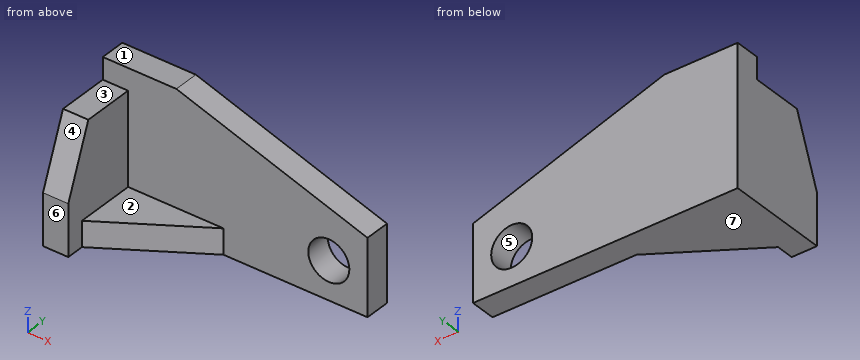
```python
from build123d import *

# Parameters (mm, degrees)
F1_DEPTH = 10.922
F3_DEPTH = 10.922
F5_DEPTH = 10.922
F6_R     = 8.859667
F7_DEPTH = 88.646


with BuildPart() as f1:
    # F0 (on Front) → F1 (new body)
    with BuildSketch(Plane.XZ):
        Polygon((31.75, 60.198), (0, 60.198), (0, 0), (114.3, 0), (114.3, 32.885686), align=None)
    extrude(amount=F1_DEPTH)

    # F2 (on Right) → F3 (join)
    with BuildSketch(Plane.YZ):
        Polygon((-44.45, 0), (0, 0), (0, 50.8), (-33.220524, 50.8), (-44.45, 22.098), align=None)
    extrude(amount=F3_DEPTH)

    # F4 (on Top) → F5 (join)
    with BuildSketch(Plane.XY):
        Polygon((52.578, -10.637136), (0, -10.637136), (0, -43.688301), align=None)
    extrude(amount=F5_DEPTH)

    # F6 (on Front) → F7 (cut)
    with BuildSketch(Plane.XZ):
        with Locations((97.587422, 16.523723)):
            Circle(F6_R)
    extrude(amount=F7_DEPTH, mode=Mode.SUBTRACT)


solid = f1.part
```
CAD build for the part. Positions are in the model's coordinates, mm. Face numbers are marked on the shaded views. A direction names the side the tool comes from. Round coordinates to 2 decimals unless told otherwise and drop trailing zeros. Write each loop counter-clockwise with the first axis right and the second up, starting at its lowest first coordinate (ties: lowest second). Pieces come first, ordered by that corner, then holes. Notation, with made-up numbers: M 64,-5 L 73,-5 A29 ccw 73,15 Z; hole C 1.25,55.5 d2. An arc over 180 degrees is marked long. One line per question, with ' | ' between items.
1. Cut at A-A on x = 93. Write the cut outline in (y, z).
Working result:
outline: M -10.92,0 L 0,0 L 0,8.94 L -10.92,8.94 Z; M -10.92,24.1 L 0,24.1 L 0,39.93 L -10.92,39.93 Z
2. Probe L1, parallel to X at y = -20.5, z = 23.5; L2, parallel to Y at x = 64, z = 3; L3, parallel to Z at x = 6, y = -22. List the from-to ranges inside material, lowest first. Write a range as from..to.
Working result:
L1: 0..10.92 | L2: -10.92..0 | L3: 0..50.8
3. Pin check, flat tips, straight feed: pin 1 Ø10 at (y, z) = (-27.5, 31) entering from +X; pin 2 Ø6 at (x, y) = (11.5, -16.5) entering from +Z; pin 3 Ø1 at (x, z) = (92.5, 42) entering from +Y; pin 4 Ø2 at (x, z) = (29.5, 7.5) entering from -Y. Stop position of each tip, or through.
Working result:
pin 1: x = 10.92 | pin 2: z = 50.8 | pin 3: through | pin 4: y = -25.77
4. Cut at C-C on y = -4. Write the cut outline in (x, z), and give its area (3 significant figures).
Working result:
outline: M 0,0 L 114.3,0 L 114.3,32.89 L 31.75,60.2 L 0,60.2 Z; hole C 97.59,16.52 d17.72 | area: 5,510 mm2
5. Cut at B-B on z = 6.5. Write the cut outline in (x, y), and give its area (3 significant figures).
Working result:
outline: M 0,-44.45 L 10.92,-44.45 L 10.92,-36.82 L 52.12,-10.92 L 114.3,-10.92 L 114.3,0 L 0,0 Z | area: 2,150 mm2
6. Mould opens along Z. For the marked faces 4, 5, 6 and 7 say: pulls with the +Z half, pulls with the -Z half, needs draft (parallel to the pull), parting line crosses it, or undercut.
Working result:
face 4: pulls with the +Z half | face 5: undercut | face 6: needs draft | face 7: pulls with the -Z half
7. Which spindle directions (+Z, -Z, +X, -X, +Y, -Y) get a long thin tool onto all of the face, cutting with end or side? Do the marked faces 1, 2 and 3. Say none if no direction does.
Working result:
face 1: +Z, +X, -X, +Y, -Y | face 2: +Z, +X, -Y | face 3: +Z, +X, -X, -Y
8. Cut at D-D on x = 40.5. Write the cut outline in (y, z), and give its area (3 significant figures).
Working result:
outline: M -18.23,0 L 0,0 L 0,57.3 L -10.92,57.3 L -10.92,10.92 L -18.23,10.92 Z | area: 706 mm2
